Work out the finished part from the listing and answer in its coordinate system (mm). Round coordinates to 2 decimals unless told otherwise and drop trailing zeros. Write each loop counter-clockwise with the first axis right and the second up, starting at its lowest first coordinate (ties: lowest second). Pieces come first, ordered by that corner, then holes. Notation, with made-up numbers: M 11,24.25 L 17,24.25 A28 cw 17,56.25 Z; hole C -1,80 d4. An arc over 180 degrees is marked long. One line per item, written item: value. Start each with the question number.
Q1. Find section B-B (y = 0). Write down the section's boundary in (x, z) (3 decimals), and give its area (3 significant figures).
Q2. Given pin 1 Ø2.5 at (x, y) = (0, 0) entering from +Z; pin 2 Ø1 at (x, z) = (-1, -1) entering from +Y, each flat-ended and moving along its own axis, determine where each tip first touches the part or whether it passes through.
Q3. Consider probe 1 along Y at (x, z) = (-0.25, -0.85); probe 2 along Y at (x, z) = (-1.5, -1.5); probe 3 along X at (y, z) = (-1.25, -2). Determine where each line is inside the solid, lowest interval first.
Q4. The mould has two halves that part along X. Classify faces 1 (the flat face through (3.5, 0, -2)), 2 (the flat face through (-2, 2, 0)), 3 (the cylindrical face through (0, -2, -2)): released by +X, released by -X, zero draft, split by the parting line, or undercut.
Q5. Find section A-A (z = -0.8). Write down the section's boundary in (x, y), and give its area (3 significant figures).
from build123d import *

# Parameters (mm, degrees)
SKETCH_1_W               = 5
SKETCH_1_H               = 3.2
SKETCH_2_OUTSIDE_W       = 14.9
SKETCH_2_OUTSIDE_H       = 14.9
CUT_EXTRUDE_1_DEPTH      = 3.2
SKETCH_3_R               = 2
CUT_EXTRUDE_2_DEPTH      = 1
CUT_EXTRUDE_2_DEPTH_BACK = 4.2
CHAMFER_1_SIZE           = 0.4


with BuildPart() as part:
    # Эскиз1 → Повернуть1 (revolve)
    with BuildSketch(Plane(origin=(0, 0, 0), x_dir=(1, 0, 0), z_dir=(0, 1, 0))):
        with Locations((-2.5, 1.6)):
            Rectangle(SKETCH_1_W, SKETCH_1_H)
    revolve(axis=Axis((0, 0, 0), (0, 0, -1)))

    # Эскиз2 outside → Вырез-Вытянуть1 (cut)
    with BuildSketch(Plane.XY):
        Rectangle(SKETCH_2_OUTSIDE_W, SKETCH_2_OUTSIDE_H)
        Polygon((3.5, -2.020725942), (3.5, 2.020725942), (0, 4.041451884), (-3.5, 2.020725942), (-3.5, -2.020725942), (0, -4.041451884), align=None, mode=Mode.SUBTRACT)
    extrude(amount=-CUT_EXTRUDE_1_DEPTH, mode=Mode.SUBTRACT)

    # Эскиз3 → Вырез-Вытянуть2 (cut, two sides)
    with BuildSketch(Plane.XY) as cut_extrude_2_sk:
        Circle(SKETCH_3_R)
    extrude(amount=CUT_EXTRUDE_2_DEPTH, mode=Mode.SUBTRACT)
    extrude(cut_extrude_2_sk.sketch, amount=-CUT_EXTRUDE_2_DEPTH_BACK, mode=Mode.SUBTRACT)

    # Эскиз4 → Вырез-Повернуть1 (revolve, cut)
    with BuildSketch(Plane(origin=(0, 0, 0), x_dir=(0, 0, -1), z_dir=(1, 0, 0))):
        Polygon((0, 3.325), (0.413643688, 4.041451884), (0, 4.041451884), align=None)
        Polygon((3.2, 3.325), (2.786356312, 4.041451884), (3.2, 4.041451884), align=None)
    revolve(axis=Axis((0, 0, 0), (0, 0, -1)), mode=Mode.SUBTRACT)

    # Фаска1
    chamfer_1_edges = [part.edges().sort_by_distance(p)[0] for p in [
        (-2, 0, -3.2),
        (-2, 0, 0),
    ]]
    chamfer(chamfer_1_edges, length=CHAMFER_1_SIZE)


solid = part.part
The answers:
1. outline: M -3.5,-3.099 L -3.325,-3.2 L -2.4,-3.2 L -2,-2.8 L -2,-0.4 L -2.4,0 L -3.325,0 L -3.5,-0.101 Z; M 2,-2.8 L 2.4,-3.2 L 3.325,-3.2 L 3.5,-3.099 L 3.5,-0.101 L 3.325,0 L 2.4,0 L 2,-0.4 Z
1. area: 9.24 mm2
2. pin 1: through
2. pin 2: y = 3.75
3. probe 1: -3.9 to -1.98, 1.98 to 3.9
3. probe 2: -3.18 to -1.32, 1.32 to 3.18
3. probe 3: -3.5 to -1.56, 1.56 to 3.5
4. face 1: released by +X
4. face 2: zero draft
4. face 3: undercut
5. outline: M -3.5,-2.02 L 0,-4.04 L 3.5,-2.02 L 3.5,2.02 L 0,4.04 L -3.5,2.02 Z; hole C 0,0 d4
5. area: 29.9 mm2
